Check sheet for the drawn part. Datum: minimum x, y, z corner. Units: mm. Give positions to 0.01 mm unless a question says otherwise; leave off trailing zeros. Write each loop counter-clockwise with the first axis right and the second up, starting at its lowest first coordinate (ties: lowest second). Pieces come first, ordered by that corner, then holes.
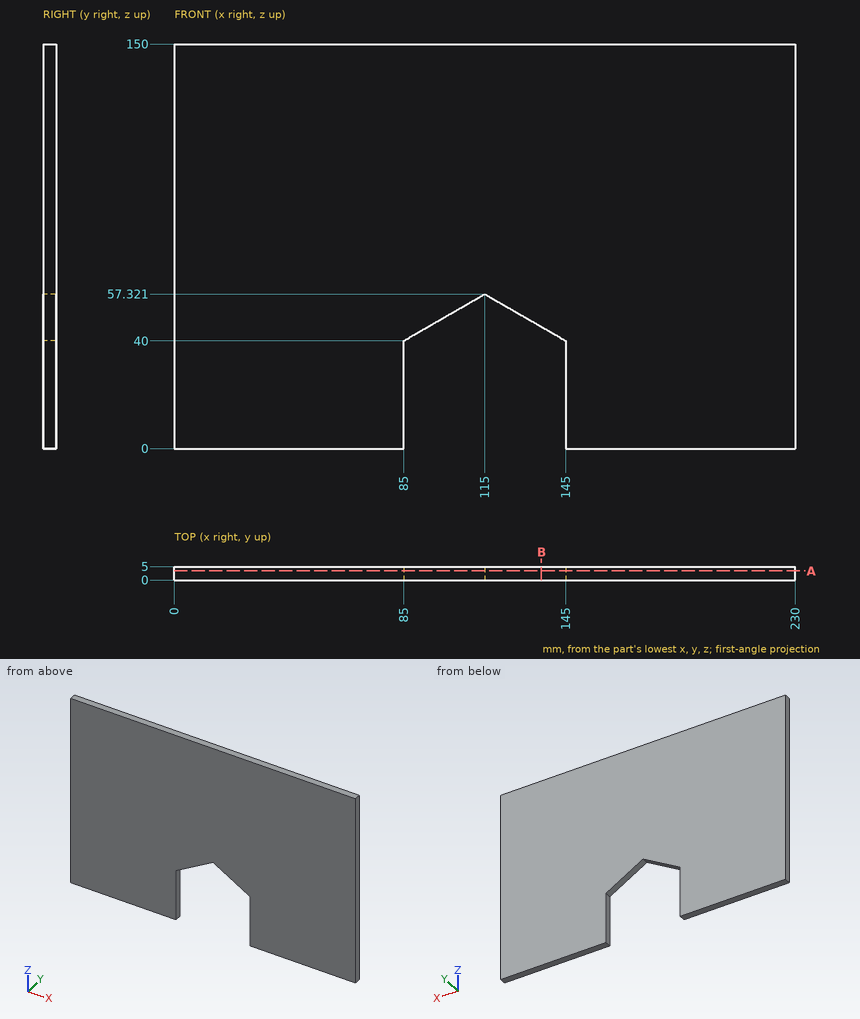
1) Sectioned sample at B-B on x = 136. Record the boundary of the cut face in (y, z), then the cut area to 3 significant figures.
2) Sectioned sample at A-A on y = 3.45. Record the boundary of the cut face in (x, z).
3) Scan lines: L1, parallel to X at y = 4.2, z = 29; L2, parallel to Z at x = 97, y = 1.1; L3, parallel to Z at x = 126.5, y = 3.4. Record each from-to range of solid material in increasing order.
Answers below:
1. outline: (0, 45.2) - (5, 45.2) - (5, 150) - (0, 150) - close
1. area: 524 mm2
2. outline: (0, 0) - (85, 0) - (85, 40) - (115, 57.32) - (145, 40) - (145, 0) - (230, 0) - (230, 150) - (0, 150) - close
3. L1: x = 0 to 85, 145 to 230
3. L2: z = 46.93 to 150
3. L3: z = 50.68 to 150
